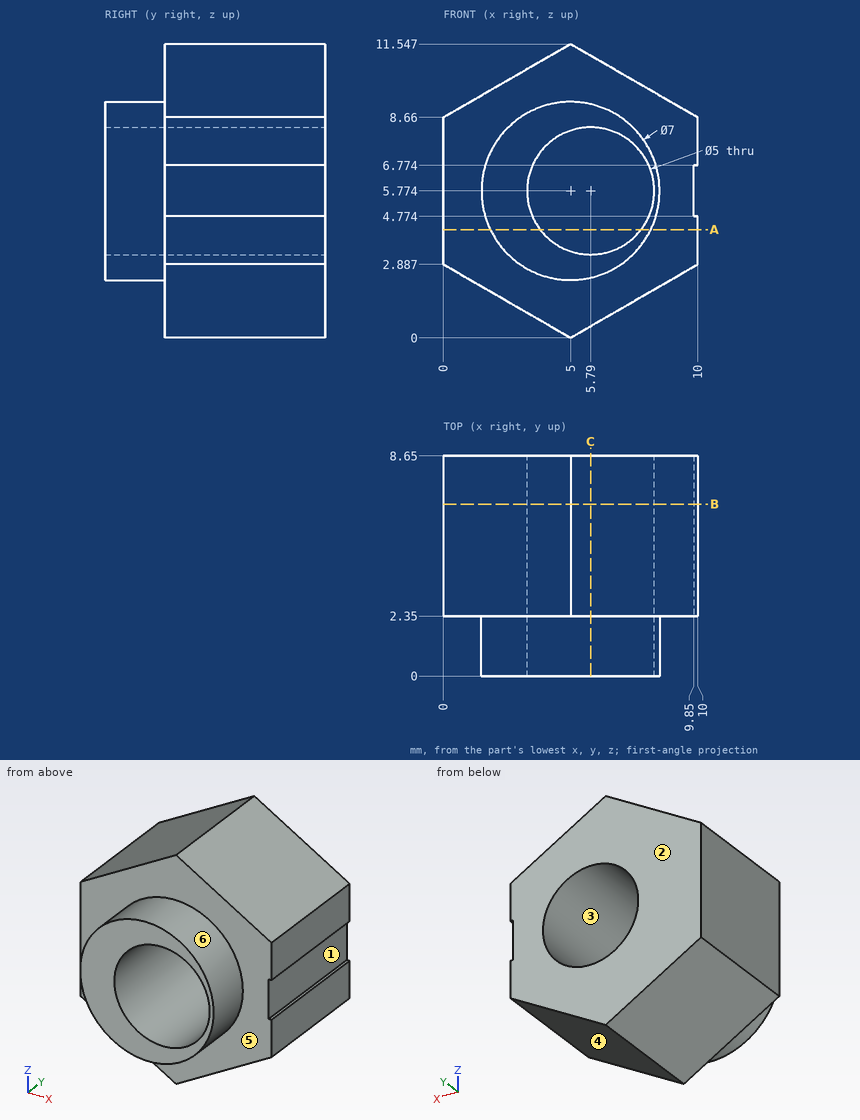
Drawing for the job (mm, zero at the part's lowest x, y, z). A direction names the side the tool comes from. Round coordinates to 2 decimals unless told otherwise and drop trailing zeros. Order: outer loops, then holes, each group sorted by start corner. A loop starts at its lowest first (then second) coordinate and runs counter-clockwise, first axis right, second up. Notation, with made-up numbers: (74.25, 49) -> (88.25, 49) arc R9 ccw to (88.25, 62) -> close; hole circle Ø6 at (-34, 38.5). An arc over 180 degrees is marked (long way). Write item = value, one per line. Start each with the question number.
(1) Cut at B-B, the plane y = 6.75. List the corners of the cut face in (x, z).
(2) Probe line 1 (Y direction, x = 9.25, z = 5); line 2 (X direction, y = 7.25, z = 5). List the from-to ranges inside material, lowest first. Write a range as [from, to].
(3) Pin check, flat tips, straight feed: P1, Ø5, axis at x = 5, z = 3.5, coming from the -Y side; P2, Ø2, axis at x = 8.5, y = 5, coming from the +Z side (1 decimal); P3, Ø0.6, axis at y = 4, z = 5.5, coming from the +X side; P4, Ø4, axis at x = 7.5, y = 3.5, coming from the +Z side. Stop position of each tip, or through.
(4) Cut at C-C, the plane x = 5.79. List the corners of the cut face in (y, z).
(5) Pull direction Z, two halves, no side cores. Call the marked faces 3, 4, 5 and 6: released by +Z, released by -Z, zero draft, split by the parting line, or undercut.
(6) Cut at A-A, the plane z = 4.25. List the corners of the cut face in (x, y).
(7) Which spindle directions (+Z, -Z, +X, -X, +Y, -Y) get a long thin tool onto all of the face, cutting with end or side? Do the marked faces 1 and 2. Say none if no direction does.
Model answer:
q1.outline = (0, 2.89) -> (5, 0) -> (10, 2.89) -> (10, 4.77) -> (9.85, 4.77) -> (9.85, 6.77) -> (10, 6.77) -> (10, 8.66) -> (5, 11.55) -> (0, 8.66) -> close; hole circle Ø5 at (5.79, 5.77)
q2.line_1 = [2.35, 8.65]
q2.line_2 = [0, 3.41], [8.17, 9.85]
q3.P1 = 0
q3.P2 = 10.1
q3.P3 = 9.85
q3.P4 = 11.26
q4.outline = (0, 2.36) -> (2.35, 2.36) -> (2.35, 0.46) -> (8.65, 0.46) -> (8.65, 3.27) -> (0, 3.27) -> close; (0, 8.27) -> (8.65, 8.27) -> (8.65, 11.09) -> (2.35, 11.09) -> (2.35, 9.18) -> (0, 9.18) -> close
q5.face_3 = undercut
q5.face_4 = released by -Z
q5.face_5 = zero draft
q5.face_6 = split by the parting line
q6.outline = (0, 2.35) -> (1.85, 2.35) -> (1.85, 0) -> (3.81, 0) -> (3.81, 8.65) -> (0, 8.65) -> close; (7.77, 0) -> (8.15, 0) -> (8.15, 2.35) -> (10, 2.35) -> (10, 8.65) -> (7.77, 8.65) -> close
q7.face_1 = +X, +Y, -Y
q7.face_2 = +Z, -Z, +X, -X, +Y
